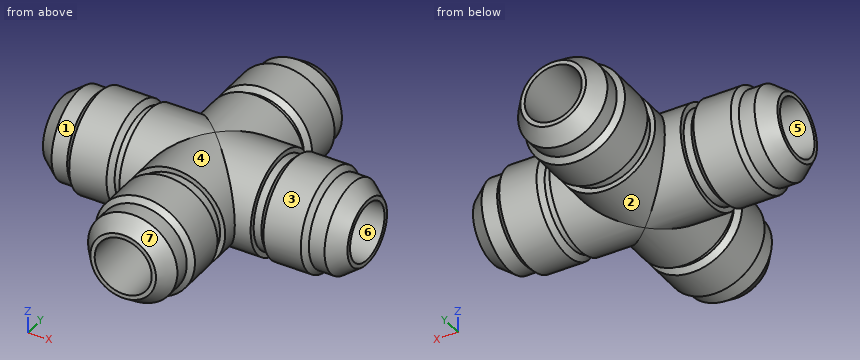
from build123d import *
from build123d.topology import SkipClean

# Parameters (mm, degrees)
SKETCH2_R               = 13.49375
EXTRUDE1_DEPTH          = 23.495
SKETCH15_R              = 13.49375
BOSS_EXTRUDE1_DEPTH     = 17.78
SKETCH16_R              = 7.7343
CUT_EXTRUDE1_DEPTH      = 46.47293924
CIRPATTERN1_COUNT       = 4
CIRPATTERN1_ANGLE       = 270
SKETCH17_R              = 7.7343
CUT_EXTRUDE2_DEPTH      = 94.274913101
CUT_EXTRUDE3_REACH      = 95.275
SKETCH18_R              = 7.7343
CUT_EXTRUDE4_DEPTH      = 60.911038679
CUT_EXTRUDE4_DEPTH_BACK = 60.911038679
SKETCH19_R              = 7.7343
CUT_EXTRUDE5_DEPTH      = 60.911038679
CUT_EXTRUDE5_DEPTH_BACK = 60.911038679
SKETCH20_R              = 7.7343


with BuildPart() as part:
    # Sketch2 → Extrude1 (new body)
    with BuildSketch(Plane(origin=(-41.275, 0, 0), x_dir=(0, 0, -1), z_dir=(1, 0, 0))):
        Circle(SKETCH2_R)
    extrude(amount=EXTRUDE1_DEPTH)

    # Sketch5 → Cut-Revolve1 (revolve, cut)
    with BuildSketch(Plane.XY):
        Polygon((-36.995957679, 12.118934671), (-32.762624346, 12.118934671), (-31.387809017, 13.49375), (-41.275, 13.49375), (-41.275, 8.894445), align=None)
        Polygon((-17.78, 12.118934671), (-19.896666667, 12.118934671), (-21.271481995, 13.49375), (-17.78, 13.49375), align=None)
    revolve(axis=Axis((0, 0, 0), (-1, 0, 0)), mode=Mode.SUBTRACT)

    # Sketch15 → Boss-Extrude1 (add)
    with BuildSketch(Plane(origin=(-17.78, 0, 0), x_dir=(0, 0, -1), z_dir=(1, 0, 0))):
        with Locations(Location((0, 0, 0), (0, 0, 90))):
            Circle(SKETCH15_R)
    extrude(amount=BOSS_EXTRUDE1_DEPTH)

    # Sketch16 → Cut-Extrude1 (cut, through all)
    with BuildSketch(Plane(origin=(0, 0, 0), x_dir=(0, 0, -1), z_dir=(1, 0, 0))):
        Circle(SKETCH16_R)
    extrude(amount=-CUT_EXTRUDE1_DEPTH, mode=Mode.SUBTRACT)


with BuildPart() as cirpattern1_1:
    # CirPattern1: pattern copy
    add(part.part.rotate(Axis((0, 0, 0), (0, 0, -1)), 1 * CIRPATTERN1_ANGLE / (CIRPATTERN1_COUNT - 1)))

    # Sketch17 → Cut-Extrude2 (cut, through all)
    with BuildSketch(Plane.ZY.offset(41.275)):
        with Locations(Location((0, 0, 0), (0, 0, 180))):
            Circle(SKETCH17_R)
    extrude(amount=-CUT_EXTRUDE2_DEPTH, mode=Mode.SUBTRACT)


with BuildPart() as cirpattern1_2:
    # CirPattern1: pattern copy
    add(part.part.rotate(Axis((0, 0, 0), (0, 0, -1)), 2 * CIRPATTERN1_ANGLE / (CIRPATTERN1_COUNT - 1)))


with BuildPart() as cirpattern1_3:
    # CirPattern1: pattern copy
    add(part.part.rotate(Axis((0, 0, 0), (0, 0, -1)), 3 * CIRPATTERN1_ANGLE / (CIRPATTERN1_COUNT - 1)))


with BuildPart() as cirpattern1_1_1:
    add(cirpattern1_1.part)

    # Combine1: union part, CirPattern1_2, CirPattern1_3
    add(part.part)
    add(cirpattern1_2.part)
    add(cirpattern1_3.part)

    # Sketch18 → Cut-Extrude3 (cut, up to next)
    with BuildSketch(Plane(origin=(0, 41.275, 0), x_dir=(1, 0, 0), z_dir=(0, 1, 0)), mode=Mode.PRIVATE) as cut_extrude3_sk1:
        with Locations(Location((0, 0, 0), (0, 0, 90))):
            Circle(SKETCH18_R)
    cut_extrude3_tool1 = extrude(cut_extrude3_sk1.sketch, amount=-CUT_EXTRUDE3_REACH, mode=Mode.PRIVATE) & cirpattern1_1_1.part
    add(cut_extrude3_tool1.solids().sort_by_distance((0, 41.275, 0))[0], mode=Mode.SUBTRACT)

    # Sketch19 → Cut-Extrude4 (cut, two sides: drawn at the far end of the back side and taken through both)
    with SkipClean():  # the faces are left unmerged after this step: merging them gives an invalid solid
        with BuildSketch(Plane(origin=(0, 0, 0), x_dir=(0, 0, -1), z_dir=(1, 0, 0)).offset(-CUT_EXTRUDE4_DEPTH_BACK)):
            Circle(SKETCH19_R)
        extrude(amount=CUT_EXTRUDE4_DEPTH + CUT_EXTRUDE4_DEPTH_BACK, mode=Mode.SUBTRACT)

    # Sketch20 → Cut-Extrude5 (cut, two sides: drawn at the far end of the back side and taken through both)
    with BuildSketch(Plane(origin=(0, 0, 0), x_dir=(1, 0, 0), z_dir=(0, 1, 0)).offset(-CUT_EXTRUDE5_DEPTH_BACK)):
        with Locations(Location((0, 0, 0), (0, 0, 90))):
            Circle(SKETCH20_R)
    extrude(amount=CUT_EXTRUDE5_DEPTH + CUT_EXTRUDE5_DEPTH_BACK, mode=Mode.SUBTRACT)


solid = cirpattern1_1_1.part
Check sheet for the modelled part. Datum: model origin and axes. Units: mm. Face numbers are marked on the shaded views. A direction names the side the tool comes from. Coordinates: 2 decimals unless noted, no trailing zeros. Write each loop counter-clockwise with the first axis right and the second up, starting at its lowest first coordinate (ties: lowest second). Pieces come first, ordered by that corner, then holes.
Item 1: Cross-section at B-B on x = -36. Record the boundary of the cut face in (y, z), then the cut area to 3 significant figures.
Numbers:
outline: circle Ø24.24 at (0, 0); hole circle Ø15.47 at (0, 0)
area: 273 mm2
Item 2: Depth check by flat-ended pin: pin 1 Ø8 at (x, z) = (-32, -8) entering from -Y; pin 2 Ø8 at (x, y) = (13, -15.5) entering from -Z; pin 3 Ø8 at (x, z) = (29.5, 3.5) entering from +Y. Enter the tip coordinate at first touch or a pass-through.
Numbers:
pin 1: stops at y = -12.87
pin 2: stops at z = -10.05
pin 3: stops at y = 13.49
Item 3: Mould release check, pull along Z, two halves, no side actions. Record for the marked faces 6 and 7: released by +Z, released by -Z, zero draft, split by the parting line, or undercut.
Numbers:
face 6: undercut
face 7: split by the parting line
Item 4: Access from +Z, -Z, +X, -X, +Y, -Y to the whole of each face (thin tool, end or side, straight path). Record for the marked faces 1, 2, 3, 4 and 5.
Numbers:
face 1: -X
face 2: +Y
face 3: +X
face 4: -Y
face 5: +X, -X
Item 5: Cross-section at C-C on z = 0. Count the separate pieces of the cut face and the enclosed holes in it, then the cut area to 3 significant figures.
Numbers:
separate pieces: 4
enclosed holes: 0
area: 1,230 mm2
Item 6: Scan lines: probe 1 along Z at (x, y) = (0, 3); probe 2 along X at (y, z) = (35, 0). Record each from-to range of solid material in increasing order.
Numbers:
probe 1: z = -13.49 to -7.73, 7.73 to 13.49
probe 2: x = -12.12 to -7.73, 7.73 to 12.12
Item 7: Cross-section at A-A on y = -15. Record the boundary of the cut face in (x, z).
Numbers:
outline: circle Ø26.99 at (0, 0); hole circle Ø15.47 at (0, 0)
